Here's how the part is built. I have some questions about the finished solid (model axes, mm). A direction names the side the tool comes from. Coordinates: 2 decimals unless noted, no trailing zeros. Write each loop counter-clockwise with the first axis right and the second up, starting at its lowest first coordinate (ties: lowest second). Pieces come first, ordered by that corner, then holes. Notation, with made-up numbers: (5, 45) - (46, 45) arc R13 cw to (46, 66) - close; hole circle Ø6 at (12.25, 1.5). An arc over 180 degrees is marked (long way). Answer in a Markdown table with one row per item. Add a question column.
Item 1: Imagine slicing it at A-A (x = 0). Please give me the cut outline in (y, z), plus the area to 3 significant figures.
Item 2: Imagine slicing it at B-B (z = 0). Please give me the cut outline in (x, y).
Item 3: Which directions (+Z, -Z, +X, -X, +Y, -Y) give clear straight access to the entire face, cutting with the end or side of a thin tool? Please do faces 1 (the face through (0, 33, 0)), 2 (the face through (3, 15, -3)), 3 (the face through (10, 0, 2)).
Item 4: Imagine slicing it at D-D (y = 21.5). Please give me the cut outline in (x, z).
Item 5: Imagine slicing it at C-C (y = 14). Please give me the cut outline in (x, z).
Item 6: If I drill on probe 1 along X at (y, z) = (-1.25, 0); probe 2 along Z at (x, y) = (-3, 0.5); probe 3 along Z at (x, y) = (10.5, 5), over which ranges is the centre line in solid material (lowest first)? Write a range as from..to.
Item 7: I'm going to push flat-ended pins straight in: pin 1 (5 mm diameter, centred on x = 8, y = -0.5, fed in from +Z); pin 2 (12 mm diameter, centred on y = 23.5, z = 0, fed in from +X); pin 3 (8 mm diameter, centred on x = -2, z = -8.5, fed in from -Y). Where does each tip first touch, or does it pass through?
from build123d import *

# Parameters (mm, degrees)
SKETCH1_R           = 12
BOSS_EXTRUDE1_DEPTH = 15
SKETCH2_R           = 4
BOSS_EXTRUDE2_DEPTH = 18
SKETCH4_R           = 8
CUT_EXTRUDE1_DEPTH  = 2
DOME1_FACE_RADIUS   = 8
DOME1_HEIGHT        = 8
SKETCH5_R           = 10.75
SKETCH5_R_2         = 7.5
BOSS_EXTRUDE3_DEPTH = 1.5
CHAMFER1_SIZE       = 2
CHAMFER1_SIZE_2     = 3.464101615


with BuildPart() as part:
    # Sketch1 → Boss-Extrude1 (new body)
    with BuildSketch(Plane(origin=(0, 0, 0), x_dir=(1, 0, 0), z_dir=(0, 1, 0))):
        with Locations(Location((0, 0, 0), (0, 0, 270))):
            Circle(SKETCH1_R)
    extrude(amount=BOSS_EXTRUDE1_DEPTH)

    # Sketch2 → Boss-Extrude2 (add)
    with BuildSketch(Plane(origin=(0, 15, 0), x_dir=(1, 0, 0), z_dir=(0, 1, 0))):
        with Locations(Location((0, 0, 0), (0, 0, 270))):
            Circle(SKETCH2_R)
    extrude(amount=BOSS_EXTRUDE2_DEPTH)

    # Sketch4 → Cut-Extrude1 (cut)
    with BuildSketch(Plane.XZ):
        with Locations(Location((0, 0, 0), (0, 0, 270))):
            Circle(SKETCH4_R)
    extrude(amount=-CUT_EXTRUDE1_DEPTH, mode=Mode.SUBTRACT)

    # Dome1: a dome of height H over a round flat face of radius A is a cap of a sphere of radius (A * A + H * H) / (2 * H)
    dome1_r = (DOME1_FACE_RADIUS * DOME1_FACE_RADIUS + DOME1_HEIGHT * DOME1_HEIGHT) / (2 * DOME1_HEIGHT)
    dome1_base = Plane((0, 2, 0), z_dir=(0, -1, 0))
    with Locations(dome1_base.offset(DOME1_HEIGHT - dome1_r)):
        dome1_ball = Sphere(dome1_r, mode=Mode.PRIVATE)
    add(split(dome1_ball, bisect_by=dome1_base, keep=Keep.TOP, mode=Mode.PRIVATE))

    # Sketch5 → Boss-Extrude3 (add)
    with BuildSketch(Plane.XZ):
        with Locations(Location((0, 0, 0), (0, 0, 90))):
            Circle(SKETCH5_R)
        with Locations(Location((0, 0, 0), (0, 0, 90))):
            Circle(SKETCH5_R_2, mode=Mode.SUBTRACT)
    extrude(amount=BOSS_EXTRUDE3_DEPTH)

    # Chamfer1
    # the kernel refuses this chamfer: 3.464101615, 2 mm, written as the material it takes off along each edge
    with BuildSketch(Plane(origin=(0, -1.5, 0), x_dir=(0, 0, 1), z_dir=(1, 0, 0))) as chamfer1_piece_1_section:
        Polygon((10.75, -CHAMFER1_SIZE), (10.75 - CHAMFER1_SIZE_2, 0), (10.75, 0), align=None)
    chamfer1_piece_1 = revolve(axis=Axis((0, -1.5, 0), (0, -1, 0)), mode=Mode.PRIVATE)
    chamfer1_piece_1 = split(chamfer1_piece_1, bisect_by=Plane(origin=(0, 0, -8.554997787), z_dir=(0, -1, 0)), keep=Keep.TOP, mode=Mode.PRIVATE)
    add(chamfer1_piece_1, mode=Mode.SUBTRACT)


solid = part.part
Here are the results:
| question | item | result |
|---|---|---|
| 1 | outline | (-1.38, -7.5) - (0, -9.88) - (0, -12) - (15, -12) - (15, -4) - (33, -4) - (33, 4) - (15, 4) - (15, 12) - (0, 12) - (0, 9.88) - (-1.38, 7.5) - (-0.78, 7.5) arc R8 ccw to (-0.78, -7.5) - close; hole (0, -8) - (2, -8) arc R8 cw to (0, -7.75) - close; hole (0, 7.75) arc R8 cw to (2, 8) - (0, 8) - close |
| 1 | area | 576 mm2 |
| 2 | outline | (-12, 0) - (-9.88, 0) - (-7.5, -1.38) - (-7.5, -0.78) arc R8 ccw to (7.5, -0.78) - (7.5, -1.38) - (9.88, 0) - (12, 0) - (12, 15) - (4, 15) - (4, 33) - (-4, 33) - (-4, 15) - (-12, 15) - close; hole (-8, 0) - (-7.75, 0) arc R8 cw to (-8, 2) - close; hole (7.75, 0) - (8, 0) - (8, 2) arc R8 cw to start |
| 3 | face 1 | +Z, -Z, +X, -X, +Y |
| 3 | face 2 | +Y |
| 3 | face 3 | -Y |
| 4 | outline | circle Ø8 at (0, 0) |
| 5 | outline | circle Ø24 at (0, 0) |
| 6 | probe 1 | x = -7.72..-7.5, -7.31..7.31, 7.5..7.72 |
| 6 | probe 2 | z = -11.62..-7.42, -7.26..7.26, 7.42..11.62 |
| 6 | probe 3 | z = -5.81..5.81 |
| 7 | pin 1 | stops at z = 10.64 |
| 7 | pin 2 | stops at x = 4 |
| 7 | pin 3 | stops at y = -4.45 |
